Check sheet for the drawn part. Datum: minimum x, y, z corner. Units: mm. Round coordinates to 2 decimals unless told otherwise and drop trailing zeros. Write each loop counter-clockwise with the first axis right and the second up, starting at its lowest first coordinate (ties: lowest second). Pieces come first, ordered by that corner, then holes. Notation, with made-up numbers: (-12, 63.25) -> (-2, 63.25) arc R20 cw to (-2, 97.25) -> close; hole circle Ø9 at (79.25, 60.25). An arc over 180 degrees is marked (long way). Use CSV: the item, a comma, the result in double quotes.
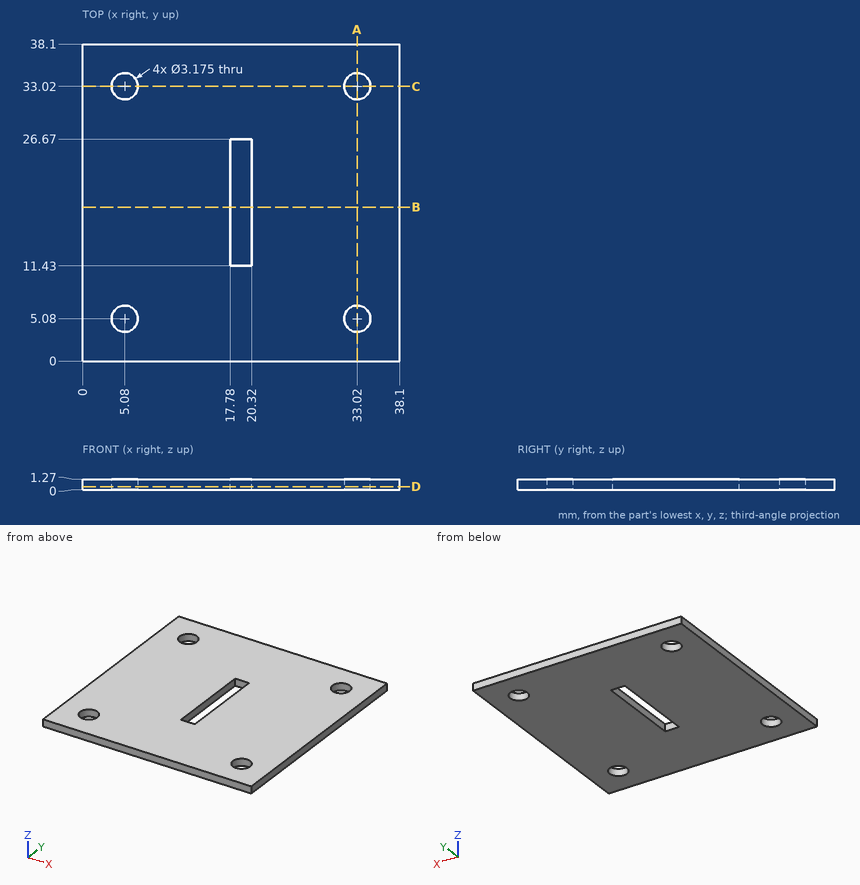
Q1. Section check A-A (x = 33.02). Record the cut outline in (y, z).
Filled in:
outline,"(0, 0) -> (3.49, 0) -> (3.49, 1.27) -> (0, 1.27) -> close; (6.67, 0) -> (31.43, 0) -> (31.43, 1.27) -> (6.67, 1.27) -> close; (34.61, 0) -> (38.1, 0) -> (38.1, 1.27) -> (34.61, 1.27) -> close"
Q2. Material ranges on L1, parallel to X at y = 5.08, z = 0.45; L2, parallel to Y at x = 20, z = 1.05, recorded low to high.
Filled in:
L1,"0 to 3.49, 6.67 to 31.43, 34.61 to 38.1"
L2,"0 to 11.43, 26.67 to 38.1"
Q3. Section check D-D (z = 0.35). Record the cut outline in (x, y) (1 decimal).
Filled in:
outline,"(0, 0) -> (38.1, 0) -> (38.1, 38.1) -> (0, 38.1) -> close; hole circle Ø3.2 at (5.1, 5.1); hole circle Ø3.2 at (5.1, 33); hole (17.8, 11.4) -> (20.3, 11.4) -> (20.3, 26.7) -> (17.8, 26.7) -> close; hole circle Ø3.2 at (33, 5.1); hole circle Ø3.2 at (33, 33)"
Q4. Section check B-B (y = 18.5). Record the cut outline in (x, z).
Filled in:
outline,"(0, 0) -> (17.78, 0) -> (17.78, 1.27) -> (0, 1.27) -> close; (20.32, 0) -> (38.1, 0) -> (38.1, 1.27) -> (20.32, 1.27) -> close"
Q5. Go/stop test with a flat-tipped pin: P1, Ø3, axis at x = 5.08, y = 33.02, coming from the -Z side (1 decimal). Record where the tip stops, or that it passes through.
Filled in:
P1,"through"
